Model file for the job. Use its own axes, mm. A direction names the side the tool comes from. Coordinates: 2 decimals unless noted, no trailing zeros. Order: outer loops, then holes, each group sorted by start corner. A loop starts at its lowest first (then second) coordinate and runs counter-clockwise, first axis right, second up.
from build123d import *


with BuildPart() as part:
    # Sketch2 → Revolve1 (revolve)
    with BuildSketch(Plane.ZY.offset(-259.301545348)):
        Polygon((4, -105.47061945), (4, -125.573704322), (46.438180449, -125.573704322), (46.438180449, -138.59916661), (42.438180449, -138.59916661), (42.438180449, -128.573704322), (0, -128.573704322), (0, -105.47061945), align=None)
    revolve(axis=Axis((259.301545348, -148.573704322, -5), (0, 0, 1)))


solid = part.part
Q1. Drop flat-ended pins along their axis: P1, Ø5, axis at x = 270.5, z = 30, coming from the -Y side; P2, Ø4, axis at x = 268, y = -154.5, coming from the -Z side; P3, Ø4, axis at y = -171, z = 21.5, coming from the -X side. Give the stop position or say it passes through.
Established:
P1: stops at y = -169.87
P2: stops at z = 42.44
P3: stops at x = 248.73
Q2. Probe line 1 (Y direction, x = 259, z = 30); line 2 (Z direction, x = 241, y = -119.5); line 3 (X direction, y = -140, z = 10). List the from-to ranges inside material, lowest first.
Established:
line 1: y = -171.57 to -168.57, -128.58 to -125.58
line 2: z = 0 to 4
line 3: x = 237.96 to 241.23, 277.37 to 280.64
Q3. Cut at D-D, the plane y = -160.5. List the corners of the cut face in (x, z).
Established:
outline: (217.88, 0) - (243.25, 0) - (243.25, 42.44) - (275.36, 42.44) - (275.36, 0) - (300.72, 0) - (300.72, 4) - (278.97, 4) - (278.97, 46.44) - (239.64, 46.44) - (239.64, 4) - (217.88, 4) - close
Q4. Cut at C-C, the plane x = 276. List the corners of the cut face in (y, z).
Established:
outline: (-188.31, 0) - (-159.58, 0) - (-159.58, 42.44) - (-137.57, 42.44) - (-137.57, 0) - (-108.84, 0) - (-108.84, 4) - (-132.76, 4) - (-132.76, 46.44) - (-164.39, 46.44) - (-164.39, 4) - (-188.31, 4) - close
Q5. Cut at A-A, the plane y = -140.5. List the corners of the cut face in (x, z).
Established:
outline: (216.96, 0) - (241, 0) - (241, 42.44) - (253.44, 42.44) - (253.44, 46.44) - (237.77, 46.44) - (237.77, 4) - (216.96, 4) - close; (265.16, 42.44) - (277.6, 42.44) - (277.6, 0) - (301.64, 0) - (301.64, 4) - (280.84, 4) - (280.84, 46.44) - (265.16, 46.44) - close
Q6. Which spindle directions (+Z, -Z, +X, -X, +Y, -Y) get a long thin tool onto all of the face, cutting with end or side? Do faces 4 (the face through (268, -167, 0)), 5 (the face through (258.422, -168.554, 20.922)). Say none if no direction does.
Established:
face 4: -Z, +X, -X, +Y, -Y
face 5: -Z
Q7. Cut at B-B, the plane x = 253. List the corners of the cut face in (y, z).
Established:
outline: (-191.21, 0) - (-167.56, 0) - (-167.56, 42.44) - (-156.31, 42.44) - (-156.31, 46.44) - (-170.69, 46.44) - (-170.69, 4) - (-191.21, 4) - close; (-140.84, 42.44) - (-129.59, 42.44) - (-129.59, 0) - (-105.93, 0) - (-105.93, 4) - (-126.45, 4) - (-126.45, 46.44) - (-140.84, 46.44) - close
Q8. Mould opens along X. For faces 1 (the face through (278, -130, 4)), 2 (the face through (243.76, -165.53, 25.52)), 3 (the face through (263, -139, 42.438)) say: pulls with the +X half, pulls with the -X half, needs draft (parallel to the pull), parting line crosses it, or undercut.
Established:
face 1: needs draft
face 2: parting line crosses it
face 3: undercut
